Autodesk Inventor part; units mm, degrees
ref_plane "C1_XY" through (0, 0, 0) normal (0, 0, 1) x (1, 0, 0)
ref_plane "C1_YZ" through (0, 0, 0) normal (1, 0, 0) x (0, 1, 0)
ref_plane "C1_ZX" through (0, 0, 0) normal (0, 1, 0) x (0, 0, 1)
sketch "Sketch_1" plane through (0, 0, 0) normal (0, 0, 1) x (1, 0, 0)
  line L0 (-15, 4) -> (-13, 4)
  line L1 (-13, 4) -> (-13, 8.25)
  line L2 (-13, 8.25) -> (-9.6642, 8.25)
  line L3 (-9.6642, 8.25) -> (-6, 4.5858)
  line L4 (-6, 4.5858) -> (-6, 0.5196)
  line L5 (-6, 0.5196) -> (-5.7, 0)
  line L6 (-5.7, 0) -> (-6, -0.5196)
  line L7 (-6, -0.5196) -> (-6, -4.5858)
  line L8 (-6, -4.5858) -> (-9.6642, -8.25)
  line L9 (-9.6642, -8.25) -> (-13, -8.25)
  line L10 (-13, -8.25) -> (-13, -4)
  line L11 (-13, -4) -> (-15, -4)
  line L12 (-15, -4) -> (-15, -13)
  arc A0 (-15, -13) -> (-13, -15) centre (-13, -13) ccw
  line L13 (-13, -15) -> (-4, -15)
  line L14 (-4, -15) -> (-4, -13)
  line L15 (-4, -13) -> (-8.25, -13)
  line L16 (-8.25, -13) -> (-8.25, -9.6642)
  line L17 (-8.25, -9.6642) -> (-4.5858, -6)
  line L18 (-4.5858, -6) -> (-0.5196, -6)
  line L19 (-0.5196, -6) -> (0, -5.7)
  line L20 (0, -5.7) -> (0.5196, -6)
  line L21 (0.5196, -6) -> (4.5858, -6)
  line L22 (4.5858, -6) -> (8.25, -9.6642)
  line L23 (8.25, -9.6642) -> (8.25, -13)
  line L24 (8.25, -13) -> (4, -13)
  line L25 (4, -13) -> (4, -15)
  line L26 (4, -15) -> (13, -15)
  arc A1 (13, -15) -> (15, -13) centre (13, -13) ccw
  line L27 (15, -13) -> (15, -4)
  line L28 (15, -4) -> (13, -4)
  line L29 (13, -4) -> (13, -8.25)
  line L30 (13, -8.25) -> (9.6642, -8.25)
  line L31 (9.6642, -8.25) -> (6, -4.5858)
  line L32 (6, -4.5858) -> (6, -0.5196)
  line L33 (6, -0.5196) -> (5.7, 0)
  line L34 (5.7, 0) -> (6, 0.5196)
  line L35 (6, 0.5196) -> (6, 4.5858)
  line L36 (6, 4.5858) -> (9.6642, 8.25)
  line L37 (9.6642, 8.25) -> (13, 8.25)
  line L38 (13, 8.25) -> (13, 4)
  line L39 (13, 4) -> (15, 4)
  line L40 (15, 4) -> (15, 13)
  arc A2 (15, 13) -> (13, 15) centre (13, 13) ccw
  line L41 (13, 15) -> (4, 15)
  line L42 (4, 15) -> (4, 13)
  line L43 (4, 13) -> (8.25, 13)
  line L44 (8.25, 13) -> (8.25, 9.6642)
  line L45 (8.25, 9.6642) -> (4.5858, 6)
  line L46 (4.5858, 6) -> (0.5196, 6)
  line L47 (0.5196, 6) -> (0, 5.7)
  line L48 (0, 5.7) -> (-0.5196, 6)
  line L49 (-0.5196, 6) -> (-4.5858, 6)
  line L50 (-4.5858, 6) -> (-8.25, 9.6642)
  line L51 (-8.25, 9.6642) -> (-8.25, 13)
  line L52 (-8.25, 13) -> (-4, 13)
  line L53 (-4, 13) -> (-4, 15)
  line L54 (-4, 15) -> (-13, 15)
  arc A3 (-13, 15) -> (-15, 13) centre (-13, 13) ccw
  line L55 (-15, 13) -> (-15, 4)
extrude "Extrusion1" add sketch "Sketch_1" against normal blind 200
sketch "Sketch2" plane through (0, 0, -200) normal (0, 0, -1) x (-1, 0, 0)
  point P0 (0, 0)
hole "Hole1" at (0, 0, -200) direction (0, 0, 1) diameter 6.8 depth 200
sketch "Sketch3" plane through (0, 0, -200) normal (0, 0, -1) x (-1, 0, 0)
  point P0 (-11.6, 11.6)
hole "Hole2" at (11.6, 11.6, -200) direction (0, 0, 1) diameter 4.2 depth 200
pattern_linear "Rectangular Pattern1" count 2 spacing 23.2 along (-1, 0, 0) count 2 spacing 23.2 along (0, -1, 0) of "Hole2"
ref_plane "C1_XY" through (0, 0, 0) normal (0, 0, 1) x (1, 0, 0)
ref_plane "C1_YZ" through (0, 0, 0) normal (1, 0, 0) x (0, 1, 0)
ref_plane "C1_ZX" through (0, 0, 0) normal (0, 1, 0) x (0, 0, 1)
ref_plane "to_frame_cap1_XY" through (0, 0, 0) normal (0, 0, 1) x (1, 0, 0)
ref_plane "to_frame_cap1_YZ" through (0, 0, 0) normal (1, 0, 0) x (0, 1, 0)
ref_plane "to_frame_cap1_ZX" through (0, 0, 0) normal (0, 1, 0) x (0, 0, 1)
ref_plane "to_frame_cap2_XY" through (0, 0, -200) normal (0, 0, -1) x (1, 0, 0)
ref_plane "to_frame_cap2_YZ" through (0, 0, -200) normal (1, 0, 0) x (0, -1, 0)
ref_plane "to_frame_cap2_ZX" through (0, 0, -200) normal (0, -1, 0) x (0, 0, -1)
properties part number "HFS6-3030-200"
Input: part model. Units: mm. Frame: model coordinates. A direction names the side the tool comes from. Give positions to 0.01 mm unless a question says otherwise; leave off trailing zeros. Write item = value, one per line. Start each with the question number.
1) Draft query along X for faces 1 (the face through (-9, -15, -99)), 2 (the face through (15, 8, -99)), 3 (the face through (6.392, -7.806, -98.6)). Return one class per face: pulls with the +X half, pulls with the -X half, needs draft (parallel to the pull), parting line crosses it, or undercut.
2) Reachability of faces 4 (the face through (-8, 15, -99)), 5 (the face through (-8.25, 11, -99)) from +Z, -Z, +X, -X, +Y, -Y: full face, straight path, thin tool, end or side. Return the list, or none.
3) Cut plane A-A (z = -63). Give the number of separate pieces and of enclosed holes in the cut face, and give its area (3 significant figures).
4) Pin query (flat end, axial travel): pin 1 (1.5 mm diameter, centred on x = 7, y = -11.5, fed in from +Z); pin 2 (0.6 mm diameter, centred on y = 14.5, z = -118, fed in from -X); pin 3 (4.5 mm diameter, centred on y = -1.5, z = -101, fed in from -X); pin 4 (4 mm diameter, centred on y = 1.5, z = -160, fed in from +X). Return the tip coordinate at first contact, or that it passes through.
5) Material intervals for L1, parallel to Y at x = 11.6, z = -63; L2, parallel to X at y = 5.5, z = -91, sorted ascending. Write a range as [from, to].
Answers follow:
q1.face_1 = needs draft
q1.face_2 = pulls with the +X half
q1.face_3 = undercut
q2.face_4 = +Z, -Z, +X, -X, +Y
q2.face_5 = +Z, -Z
q3.separate_pieces = 1
q3.enclosed_holes = 5
q3.area = 332 mm^2
q4.pin_1 = through
q4.pin_2 = -14.6
q4.pin_3 = -6
q4.pin_4 = 6
q5.L1 = [-15, -13.7], [-9.5, -8.25], [8.25, 9.5], [13.7, 15]
q5.L2 = [-15, -13], [-6.91, 6.91], [13, 15]
